from build123d import *

# Parameters (mm, degrees)
SKETCH1_W           = 13
SKETCH1_H           = 5.6
BOSS_EXTRUDE1_DEPTH = 6
SKETCH2_R           = 0.4
SKETCH2_W           = 0.7
SKETCH2_H           = 2.2
BOSS_EXTRUDE2_DEPTH = 3
SKETCH3_W           = 5.9
SKETCH3_H           = 3.5
BOSS_EXTRUDE3_DEPTH = 3


with BuildPart() as part:
    # Sketch1 → Boss-Extrude1 (new body)
    with BuildSketch(Plane(origin=(0, 0, 0), x_dir=(1, 0, 0), z_dir=(0, 1, 0))):
        Rectangle(SKETCH1_W, SKETCH1_H)
    extrude(amount=BOSS_EXTRUDE1_DEPTH)

    # Sketch2 → Boss-Extrude2 (add)
    with BuildSketch(Plane(origin=(0, 6, 0), x_dir=(1, 0, 0), z_dir=(0, 1, 0))):
        with Locations(Location((-3, 0, 0), (0, 0, 270))):
            Circle(SKETCH2_R)
        with Locations(Location((0, 0, 0), (0, 0, 270))):
            Circle(SKETCH2_R)
        with Locations(Location((3, 0, 0), (0, 0, 270))):
            Circle(SKETCH2_R)
        with Locations((-6.15, 0)):
            Rectangle(SKETCH2_W, SKETCH2_H)
        with Locations((6.15, 0)):
            Rectangle(SKETCH2_W, SKETCH2_H)
    extrude(amount=BOSS_EXTRUDE2_DEPTH)

    # Sketch3 → Boss-Extrude3 (add)
    with BuildSketch(Plane.XY.offset(2.8)):
        with Locations((0, 3)):
            Rectangle(SKETCH3_W, SKETCH3_H)
    extrude(amount=BOSS_EXTRUDE3_DEPTH)


solid = part.part
Can you work these out from the model? Positions are in its coordinate system, mm. A direction names the side the tool comes from. Coordinates: 2 decimals unless noted, no trailing zeros. Write each loop counter-clockwise with the first axis right and the second up, starting at its lowest first coordinate (ties: lowest second). Pieces come first, ordered by that corner, then holes. Notation, with made-up numbers: M -13.75,19.5 L 45.25,19.5 A24 ccw 45.25,55.5 Z; hole C 61.25,-39 d8. An arc over 180 degrees is marked long. Use one line per item in the form item = value.
Q1. If we section it at B-B (z = 0): Write out the boundary of the cut face in (x, y).
Model answer:
outline = M -6.5,0 L 6.5,0 L 6.5,9 L 5.8,9 L 5.8,6 L 3.4,6 L 3.4,9 L 2.6,9 L 2.6,6 L 0.4,6 L 0.4,9 L -0.4,9 L -0.4,6 L -2.6,6 L -2.6,9 L -3.4,9 L -3.4,6 L -5.8,6 L -5.8,9 L -6.5,9 Z
Q2. I need wall thicknesses on line 1 along X through (y, z) = (7.5, 0.75); line 2 along Y through (x, z) = (-4.75, 0.25); line 3 along Y through (x, z) = (2.25, 4.5). Which ranges of each line are inside material? Lowest first, please. Write a range as from..to.
Model answer:
line_1 = -6.5..-5.8, 5.8..6.5
line_2 = 0..6
line_3 = 1.25..4.75
Q3. If we section it at C-C (x = 0): Write out the boundary of the cut face in (y, z), then the cut area to 3 significant figures.
Model answer:
outline = M 0,-2.8 L 6,-2.8 L 6,-0.4 L 9,-0.4 L 9,0.4 L 6,0.4 L 6,2.8 L 4.75,2.8 L 4.75,5.8 L 1.25,5.8 L 1.25,2.8 L 0,2.8 Z
area = 46.5 mm^2
Q4. For P1, Ø1.5, axis at y = 2.5, z = 4.5, coming from the +X side; P2, Ø0.8, axis at x = 6.5, y = 7.5, coming from the +Z side; P3, Ø0.6, axis at x = -6, y = 7.5, coming from the -Z side, each with a flat end and sliding along its axis, tell me the tip position at first contact or that it passes through.
Model answer:
P1 = 2.95
P2 = 1.1
P3 = -1.1
Q5. We'd pull the mould along X, two halves only. Please class faces 1 (the flat face through (6.5, 3, 0)), 2 (the flat face through (5.8, 7, 0)), 3 (the flat face through (0, 1, 2.8)): +X half, -X half, draft (parallel to the pull), parting line (faces both ways), or undercut.
Model answer:
face_1 = +X half
face_2 = undercut
face_3 = draft
Q6. If we section it at A-A (y = 8): Write out the boundary of the cut face in (x, z).
Model answer:
outline = M -6.5,-1.1 L -5.8,-1.1 L -5.8,1.1 L -6.5,1.1 Z; C -3,0 d0.8; C 0,0 d0.8; C 3,0 d0.8; M 5.8,-1.1 L 6.5,-1.1 L 6.5,1.1 L 5.8,1.1 Z
Q7. If we section it at D-D (y = 1.5): Write out the boundary of the cut face in (x, z), then the cut area to 3 significant figures.
Model answer:
outline = M -6.5,-2.8 L 6.5,-2.8 L 6.5,2.8 L 2.95,2.8 L 2.95,5.8 L -2.95,5.8 L -2.95,2.8 L -6.5,2.8 Z
area = 90.5 mm^2
Q8. For faces 4 (the flat face through (0, 4.75, 4)), 5 (the flat face through (-5.8, 7, 0)), 6 (the flat face through (0, 1.25, 4)), 7 (the flat face through (-2.95, 3, 4)), 8 (the flat face through (2.95, 3, 4)), which set-ups out of +Z, -Z, +X, -X, +Y, -Y let a thin tool reach every point of the face, with its end or its side?
Model answer:
face_4 = +Z, +X, -X, +Y
face_5 = +Z, -Z, +Y
face_6 = +Z, +X, -X, -Y
face_7 = +Z, -X, +Y, -Y
face_8 = +Z, +X, +Y, -Y
